from build123d import *

# Parameters (mm, degrees)
F2_SIZE = 1
F3_R    = 1


with BuildPart() as f1:
    # F0 (on Right) → F1 (revolve)
    with BuildSketch(Plane.YZ):
        Polygon((0, 7.2), (0, 0), (19, 0), (19, 3.005), (35, 3.005), (35, 11), (10, 11), (10, 7.2), align=None)
    revolve(axis=Axis((0, 9.5, 0), (0, -1, 0)))

    # F2
    f2_edges = [f1.edges().sort_by_distance(p)[0] for p in [
        (0, 0, -7.2),
        (0, 10, -11),
        (0, 35, -11),
        (0, 35, -3.005),
    ]]
    chamfer(f2_edges, length=F2_SIZE)

    # F3
    f3_edges = [f1.edges().sort_by_distance(p)[0] for p in [
        (0, 10, -7.2),
    ]]
    fillet(f3_edges, radius=F3_R)


solid = f1.part
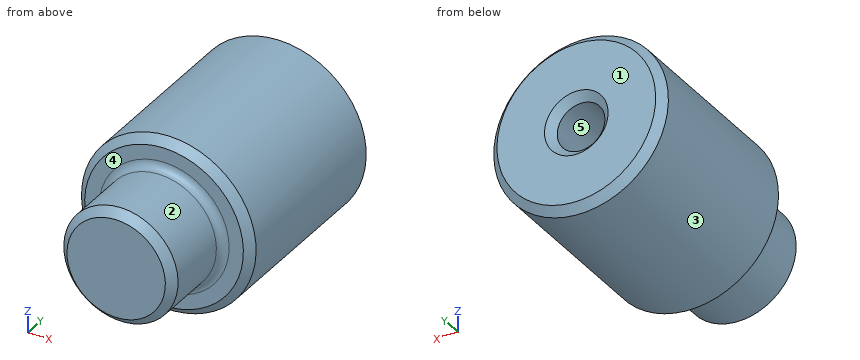
Can you work these out from the model? Positions are in its coordinate system, mm. Face numbers are marked on the shaded views. A direction names the side the tool comes from. Coordinates: 2 decimals unless noted, no trailing zeros. Write each loop counter-clockwise with the first axis right and the second up, starting at its lowest first coordinate (ties: lowest second). Pieces come first, ordered by that corner, then holes. Notation, with made-up numbers: (-6, 17.25) -> (11, 17.25) arc R16 cw to (11, 23.25) -> close; hole circle Ø1 at (-39, 41). An arc over 180 degrees is marked (long way). Write each question's results on one line, items separated by ' | '. Start each with the question number.
Q1. We'd pull the mould along Z, two halves only. Please class the marked faces 3, 4 and 5: +Z half, -Z half, draft (parallel to the pull), parting line (faces both ways), or undercut.
Q2. Imagine slicing it at B-B (x = 0). Write out the boundary of the cut face in (y, z) (3 decimals).
Q3. Imagine slicing it at A-A (z = 0). Write out the boundary of the cut face in (x, y) (3 decimals), then the cut area to 3 significant figures.
Q4. On a 3-axis mill with a long thin cutter (end or side, diameter ignored), from which of +Z, -Z, +X, -X, +Y, -Y can I reach the whole of each face in a straight line? I mean the marked faces 1 and 2. Say none if no direction works.
Q5. Imagine slicing it at D-D (y = 17). Write out the boundary of the cut face in (x, z).
Q6. I'm going to push flat-ended pins straight in: pin 1 (2 mm diameter, centred on x = 3.5, y = 21, fed in from -Z); pin 2 (1.5 mm diameter, centred on x = 7.5, z = -2.5, fed in from -Y); pin 3 (2 mm diameter, centred on x = 3.5, y = 30.5, fed in from +Z). Where does each tip first touch, or does it pass through?
Q7. If I drill on probe 1 along X at (y, z) = (28.25, 0) (3 decimals); probe 2 along Y at (x, z) = (8.25, -2.75), over which ranges is the centre line in solid material (lowest first)?
Q8. Imagine slicing it at C-C (y = 25). Write out the boundary of the cut face in (x, z) (3 decimals), then the cut area to 3 significant figures.
Taken from the geometry:
1) face 3: parting line | face 4: draft | face 5: undercut
2) outline: (0, -6.2) -> (1, -7.2) -> (9, -7.2) arc R1 cw to (10, -8.2) -> (10, -10) -> (11, -11) -> (34, -11) -> (35, -10) -> (35, -4.005) -> (34, -3.005) -> (19, -3.005) -> (19, 3.005) -> (34, 3.005) -> (35, 4.005) -> (35, 10) -> (34, 11) -> (11, 11) -> (10, 10) -> (10, 8.2) arc R1 cw to (9, 7.2) -> (1, 7.2) -> (0, 6.2) -> close
3) outline: (-11, 11) -> (-10, 10) -> (-8.2, 10) arc R1 cw to (-7.2, 9) -> (-7.2, 1) -> (-6.2, 0) -> (6.2, 0) -> (7.2, 1) -> (7.2, 9) arc R1 cw to (8.2, 10) -> (10, 10) -> (11, 11) -> (11, 34) -> (10, 35) -> (4.005, 35) -> (3.005, 34) -> (3.005, 19) -> (-3.005, 19) -> (-3.005, 34) -> (-4.005, 35) -> (-10, 35) -> (-11, 34) -> close | area: 594 mm^2
4) face 1: +Z, -Z, +X, -X, +Y | face 2: -Y
5) outline: circle Ø22 at (0, 0)
6) pin 1: stops at z = -10.71 | pin 2: stops at y = 0.96 | pin 3: stops at z = 10.71
7) probe 1: x = -11 to -3.005, 3.005 to 11 | probe 2: y = 10 to 35
8) outline: circle Ø22 at (0, 0); hole circle Ø6.01 at (0, 0) | area: 352 mm^2
